Could you check a few things on this model? Use its own coordinates, in mm. A direction names the side the tool comes from. Coordinates: 2 decimals unless noted, no trailing zeros. Answer as CSV lines item,"result". Start each with the question number.
Item 1: I'm going to push flat-ended pins straight in: P1, Ø5, axis at x = 33, y = 23.5, coming from the -Z side; P2, Ø2, axis at x = -27, y = 31.5, coming from the -Z side; P3, Ø13.5, axis at y = 29.5, z = 54, coming from the -X side; P4, Ø3, axis at x = 30, z = -30, coming from the -Y side. Where does each tip first touch, or does it pass through?
Item 2: On a 3-axis mill with a long thin cutter (end or side, diameter ignored), from which of +Z, -Z, +X, -X, +Y, -Y can I reach the whole of each face in a straight line? I mean faces 1 (the flat face through (-27, 74, 40)), 2 (the flat face through (-1, 76.125, -21)), 3 (the cylindrical face through (19, 49, 74)). Say none if no direction works.
Item 3: We'd pull the mould along Y, two halves only. Please class faces 4 (the flat face through (-11, 71.125, -11)), 5 (the flat face through (-35, 39, -24)), 6 (the flat face through (-35, 39, 24)), 7 (the cylindrical face through (-37.15, 2.54, -36.99)): +Y half, -Y half, draft (parallel to the pull), parting line (faces both ways), or undercut.
Item 4: If I drill on line 1 along X through (y, z) = (3.05, 30); line 2 along X through (y, z) = (42, 59.5); line 3 along Y through (x, z) = (-27, 34) (3 decimals), over which ranges is the centre line in solid material (lowest first)? Write a range as [from, to].
```python
from build123d import *

# Parameters (mm, degrees)
SKETCH1_W                       = 80
SKETCH1_H                       = 40
BOSS_EXTRUDE1_DEPTH             = 76.125
FILLET1_R                       = 10
CUT_EXTRUDE1_START              = -66.125
CUT_EXTRUDE1_DEPTH              = 66.125
SKETCH5_R                       = 2.5
CUT_EXTRUDE2_DEPTH              = 95.842056369
SKETCH6_R                       = 20
CUT_EXTRUDE3_DEPTH              = 5
SKETCH7_W                       = 20
SKETCH7_H                       = 40
BOSS_EXTRUDE3_DEPTH             = 76.125
FILLET2_R                       = 10
MIRROR2_START                   = -66.125
MIRROR2_COPY_1_DEPTH            = 66.125
BOSS_EXTRUDE4_REACH             = 96.842
BOSS_EXTRUDE4_DIRECTION_2_REACH = 96.842
CUT_EXTRUDE4_REACH              = 96.842
SKETCH12_R                      = 10.5
SKETCH13_W                      = 4
SKETCH13_H                      = 76.125
BOSS_EXTRUDE5_DEPTH             = 40
BOSS_EXTRUDE6_REACH             = 127.678
BOSS_EXTRUDE7_REACH             = 119.452
SKETCH15_W                      = 40
SKETCH15_H                      = 4
FILLET3_R                       = 5


with BuildPart() as part:
    # Sketch1 → Boss-Extrude1 (new body)
    with BuildSketch(Plane(origin=(0, 0, 0), x_dir=(1, 0, 0), z_dir=(0, 1, 0))):
        with Locations((0, 20)):
            Rectangle(SKETCH1_W, SKETCH1_H)
    extrude(amount=BOSS_EXTRUDE1_DEPTH)

    # Cut-Loft1: read off the stored shape, not the designer's step
    # Cut-Loft1: loft between two sections, ruled curve by curve
    cut_loft1_from = [
        Edge.make_bspline([(-2.197461017, 76.125, 14.838165826), (-31.873792669, 76.125, 10.443243791), (-27.478870634, 76.125, -19.233087861), (2.197461017, 76.125, -14.838165826), (31.873792669, 76.125, -10.443243791), (27.478870634, 76.125, 19.233087861), (-2.197461017, 76.125, 14.838165826)], [0, 0, 0, 0, 0.5, 0.5, 0.5, 1, 1, 1, 1], 3, [1, 0.333333333, 0.333333333, 1, 0.333333333, 0.333333333, 1]),
    ]
    cut_loft1_to = [
        Edge.make_bspline([(1.080050789, 0, 10.444304203), (-19.808557618, 0, 12.604405781), (-21.968659196, 0, -8.284202626), (-1.080050789, 0, -10.444304203), (19.808557618, 0, -12.604405781), (21.968659196, 0, 8.284202626), (1.080050789, 0, 10.444304203)], [0, 0, 0, 0, 0.5, 0.5, 0.5, 1, 1, 1, 1], 3, [1, 0.333333333, 0.333333333, 1, 0.333333333, 0.333333333, 1]),
    ]
    cut_loft1 = Solid(Shell([*[Face.make_surface_from_curves(cut_loft1_from[k], cut_loft1_to[k]) for k in range(1)], Face(Wire(cut_loft1_from)), Face(Wire(cut_loft1_to))]))
    add(cut_loft1, mode=Mode.SUBTRACT)

    # Fillet1
    fillet1_edges = [part.edges().sort_by_distance(p)[0] for p in [
        (-40, 38.0625, -40),
        (40, 38.0625, -40),
    ]]
    fillet(fillet1_edges, radius=FILLET1_R)

    # Sketch4 → Cut-Extrude1 (cut)
    with BuildSketch(Plane(origin=(0, 5, 0), x_dir=(-1, 0, 0), z_dir=(0, -1, 0)).offset(CUT_EXTRUDE1_START)):
        with BuildLine():
            Line((-40, 24), (-40, 30))
            ThreePointArc((-40, 30), (-37.071067812, 37.071067812), (-30, 40))
            Line((-30, 40), (-24, 40))
            Line((-24, 40), (-24, 30))
            ThreePointArc((-24, 30), (-25.757359313, 25.757359313), (-30, 24))
            Line((-30, 24), (-40, 24))
        make_face()
    cut_extrude1 = extrude(amount=CUT_EXTRUDE1_DEPTH, mode=Mode.SUBTRACT)

    # Sketch5 → Cut-Extrude2 (cut, through all)
    with BuildSketch(Plane(origin=(0, 76.125, 0), x_dir=(1, 0, 0), z_dir=(0, 1, 0))):
        with Locations(Location((30, 30, 0), (0, 0, 270))):
            Circle(SKETCH5_R)
        with Locations(Location((-30, 30, 0), (0, 0, 270))):
            Circle(SKETCH5_R)
    cut_extrude2 = extrude(amount=-CUT_EXTRUDE2_DEPTH, mode=Mode.SUBTRACT)

    # Sketch6 → Cut-Extrude3 (cut)
    with BuildSketch(Plane(origin=(0, 76.125, 0), x_dir=(1, 0, 0), z_dir=(0, 1, 0))):
        Circle(SKETCH6_R)
    extrude(amount=-CUT_EXTRUDE3_DEPTH, mode=Mode.SUBTRACT)

    # Mirror1: Cut-Extrude1 across plane
    add(cut_extrude1.mirror(Plane(origin=(0, 0, 0), x_dir=(0, 0, 1), z_dir=(1, 0, 0))), mode=Mode.SUBTRACT)

    # Sketch7 → Boss-Extrude3 (add)
    with BuildSketch(Plane(origin=(0, 76.125, 0), x_dir=(1, 0, 0), z_dir=(0, 1, 0))):
        with Locations((-30, -20)):
            Rectangle(SKETCH7_W, SKETCH7_H)
        with Locations((30, -20)):
            Rectangle(SKETCH7_W, SKETCH7_H)
    extrude(amount=-BOSS_EXTRUDE3_DEPTH)

    # Fillet2
    fillet2_edges = [part.edges().sort_by_distance(p)[0] for p in [
        (-40, 38.0625, 40),
        (40, 38.0625, 40),
    ]]
    fillet(fillet2_edges, radius=FILLET2_R)

    # Mirror2: Cut-Extrude1, Cut-Extrude2 across plane
    add(cut_extrude1.mirror(Plane.XY), mode=Mode.SUBTRACT)
    add(cut_extrude2.mirror(Plane.XY), mode=Mode.SUBTRACT)

    # Mirror2 copy 1 sketch → Mirror2 copy 1 (cut)
    with BuildSketch(Plane.XZ.offset(-5).offset(MIRROR2_START)):
        with BuildLine():
            Line((-40, 24), (-40, 30))
            ThreePointArc((-40, 30), (-37.071067812, 37.071067812), (-30, 40))
            Line((-30, 40), (-24, 40))
            Line((-24, 40), (-24, 30))
            ThreePointArc((-24, 30), (-25.757359313, 25.757359313), (-30, 24))
            Line((-30, 24), (-40, 24))
        make_face()
    extrude(amount=MIRROR2_COPY_1_DEPTH, mode=Mode.SUBTRACT)

    # Sketch9 → Loft1 section 0
    with BuildSketch(Plane.XZ):
        with BuildLine():
            Line((20, 40), (20, 0))
            Line((20, 0), (10.5, 0))
            Line((10.5, 0), (20, 40))
        make_face()
    # Sketch8 → Loft1 section 1
    with BuildSketch(Plane(origin=(0, 71.125, 0), x_dir=(1, 0, 0), z_dir=(0, 1, 0))):
        with BuildLine():
            Line((14.683973591, 0), (20, -40))
            Line((20, -40), (20, 0))
            Line((20, 0), (14.683973591, 0))
        make_face()
    loft1 = loft()

    # Mirror3: Loft1 across plane
    add(loft1.mirror(Plane(origin=(0, 0, 0), x_dir=(0, 0, 1), z_dir=(1, 0, 0))))

    # Sketch11 → Boss-Extrude4 (add, up to next)
    with BuildSketch(Plane(origin=(0, 0, 0), x_dir=(0, 0, -1), z_dir=(1, 0, 0)), mode=Mode.PRIVATE) as boss_extrude4_sk1:
        Polygon((0, 0), (-40, 0), (-40, 10), (0, 0.5), align=None)
    boss_extrude4_tool1 = extrude(boss_extrude4_sk1.sketch, amount=BOSS_EXTRUDE4_REACH, mode=Mode.PRIVATE) - part.part
    add(boss_extrude4_tool1.solids().sort_by_distance((0, 3.34127, 26.031746))[0])

    # Sketch11 → Boss-Extrude4 direction 2 (add, up to next)
    with BuildSketch(Plane(origin=(0, 0, 0), x_dir=(0, 0, -1), z_dir=(1, 0, 0)), mode=Mode.PRIVATE) as boss_extrude4_direction_2_sk1:
        Polygon((0, 0), (-40, 0), (-40, 10), (0, 0.5), align=None)
    boss_extrude4_direction_2_tool1 = extrude(boss_extrude4_direction_2_sk1.sketch, amount=-BOSS_EXTRUDE4_DIRECTION_2_REACH, mode=Mode.PRIVATE) - part.part
    add(boss_extrude4_direction_2_tool1.solids().sort_by_distance((0, 3.34127, 26.031746))[0])

    # Sketch12 → Cut-Extrude4 (cut, up to next)
    with BuildSketch(Plane(origin=(0, 0, 0), x_dir=(-1, 0, 0), z_dir=(0, -1, 0)), mode=Mode.PRIVATE) as cut_extrude4_sk1:
        Circle(SKETCH12_R)
    cut_extrude4_tool1 = extrude(cut_extrude4_sk1.sketch, amount=-CUT_EXTRUDE4_REACH, mode=Mode.PRIVATE) & part.part
    add(cut_extrude4_tool1.solids().sort_by_distance((0, 0, 0))[0], mode=Mode.SUBTRACT)

    # Sketch13 → Boss-Extrude5 (add)
    with BuildSketch(Plane.XY.offset(40)):
        with Locations((-22, 38.0625)):
            Rectangle(SKETCH13_W, SKETCH13_H)
    boss_extrude5 = extrude(amount=BOSS_EXTRUDE5_DEPTH)

    # Mirror4: Boss-Extrude5 across plane
    add(boss_extrude5.mirror(Plane(origin=(0, 0, 0), x_dir=(0, 0, 1), z_dir=(1, 0, 0))))

    # Sketch14 → Boss-Extrude6 (add, up to next)
    with BuildSketch(Plane(origin=(-20, 0, 0), x_dir=(0, 0, -1), z_dir=(1, 0, 0)), mode=Mode.PRIVATE) as boss_extrude6_sk1:
        Polygon((-40, 10), (-80, 19.5), (-80, 0), (-40, 0), align=None)
    boss_extrude6_tool1 = extrude(boss_extrude6_sk1.sketch, amount=BOSS_EXTRUDE6_REACH, mode=Mode.PRIVATE) - part.part
    add(boss_extrude6_tool1.solids().sort_by_distance((-20, 7.629944, 62.146893))[0])

    # Boss-Extrude7: up to this plane
    boss_extrude7_end = Plane(origin=(-500000, 0.5, 0), z_dir=(0, 0.9729365507195606, -0.23107243079589554))
    # Sketch15 → Boss-Extrude7 (add, up to the surface)
    with BuildSketch(Plane(origin=(0, 76.125, 0), x_dir=(1, 0, 0), z_dir=(0, 1, 0)), mode=Mode.PRIVATE) as boss_extrude7_sk1:
        with Locations((0, -78)):
            Rectangle(SKETCH15_W, SKETCH15_H)
    boss_extrude7_tool1 = split(extrude(boss_extrude7_sk1.sketch, amount=-BOSS_EXTRUDE7_REACH, mode=Mode.PRIVATE), bisect_by=boss_extrude7_end, keep=Keep.BOTH, mode=Mode.PRIVATE)
    add(boss_extrude7_tool1.solids().sort_by_distance((0, 76.125, 78))[0])

    # Fillet3
    fillet3_edges = [part.edges().sort_by_distance(p)[0] for p in [
        (-20, 40.5625, 40),
        (20, 40.5625, 40),
        (-24, 38.0625, 80),
        (24, 38.0625, 80),
        (-20, 14.275, 58),
        (20, 14.275, 58),
        (0, 18.55, 76),
        (-20, 47.3375, 76),
        (20, 47.3375, 76),
    ]]
    fillet(fillet3_edges, radius=FILLET3_R)


solid = part.part
```
Ans:
1,P1,"stops at z = -24"
1,P2,"stops at z = -25.53"
1,P3,"stops at x = -24"
1,P4,"passes through"
2,face 1,"+Z, -X, +Y, -Y"
2,face 2,"+Z, -Z, +X, -X, +Y"
2,face 3,"+Y"
3,face 4,"+Y half"
3,face 5,"undercut"
3,face 6,"undercut"
3,face 7,"draft"
4,line 1,"x = [-40, -32.5], [-27.5, 27.5], [32.5, 40]"
4,line 2,"x = [-24, -20], [20, 24]"
4,line 3,"y = [0, 5], [71.125, 76.125]"
